Part model, mm, in its own coordinate system. Face numbers are marked on the shaded views. A direction names the side the tool comes from. Round coordinates to 2 decimals unless told otherwise and drop trailing zeros. Write each loop counter-clockwise with the first axis right and the second up, starting at its lowest first coordinate (ties: lowest second). Pieces come first, ordered by that corner, then holes. Notation, with made-up numbers: (40.5, -7.5) -> (77.5, -7.5) arc R22 cw to (77.5, 7.5) -> close; hole circle Ø5 at (69, -29). An arc over 180 degrees is marked (long way). Return JSON: item names as keys, results as strings. Group by question number.
(1) Drop flat-ended pins along their axis: pin 1 Ø2 at (x, z) = (7.5, -2) entering from -Y; pin 2 Ø8 at (x, y) = (6, 38.5) entering from -Z. Give the stop position or say it passes through.
(2) Tool access for the marked faces 1 and 2: list every direction of +Z, -Z, +X, -X, +Y, -Y with a clear straight run to the whole face (end or side of a thin tool).
(3) Saw through at B-B (x = 0). List the corners of the cut face in (y, z), plus the area to 3 significant figures.
(4) Mould opens along Y. For the marked faces 3, 4 and 5 say: +Y half, -Y half, draft (parallel to the pull), parting line (faces both ways), or undercut.
(5) Saw through at A-A (x = 7.5). State how many separate pieces and enclosed holes the cut face has, plus the area to 3 significant figures.
(6) Drill centre lines: L1, parallel to Y at x = 3, z = -3.25; L2, parallel to X at y = 5.5, z = -2; L3, parallel to Z at x = -7.5, y = 85.45. Where is each one in solid material? Low to high. Write a range as from..to.
(7) Saw through at D-D (y = 21). List the corners of the cut face in (x, z), plus the area to 3 significant figures.
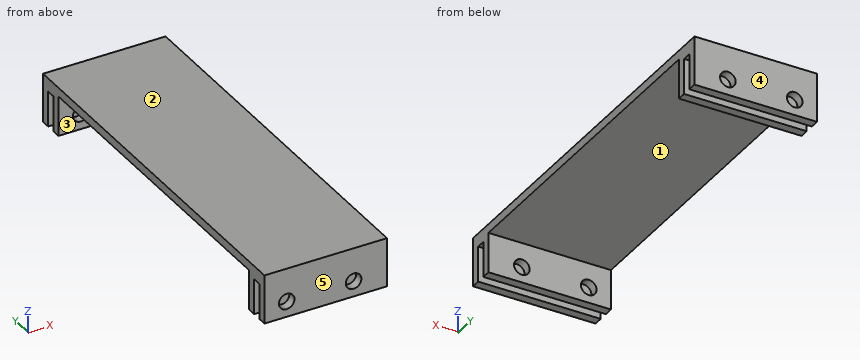
from build123d import *

# Parameters (mm, degrees)
SKETCH_1_W          = 30
SKETCH_1_H          = 11
EXTRUDE_1_DEPTH     = 6
SKETCH_2_W          = 16
SKETCH_2_H          = 2
CUT_EXTRUDE_1_DEPTH = 144
EXTRUDE_2_DEPTH     = 74
SKETCH_4_R          = 1.75
CUT_EXTRUDE_2_DEPTH = 144
SKETCH_5_W          = 11
SKETCH_5_H          = 80
CUT_EXTRUDE_3_DEPTH = 2.5
SKETCH_7_W          = 4
SKETCH_7_H          = 9
CUT_EXTRUDE_4_DEPTH = 74


with BuildPart() as part:
    # 草图1 → 凸台-拉伸1 (new body)
    with BuildSketch(Plane(origin=(0, 0, 0), x_dir=(1, 0, 0), z_dir=(0, 1, 0))):
        Rectangle(SKETCH_1_W, SKETCH_1_H)
    extrude_1 = extrude(amount=EXTRUDE_1_DEPTH)

    # 草图2 → 切除-拉伸1 (cut)
    with BuildSketch(Plane.ZY.offset(15)):
        with Locations((-5.5, 3)):
            Rectangle(SKETCH_2_W, SKETCH_2_H)
    cut_extrude_1 = extrude(amount=-CUT_EXTRUDE_1_DEPTH, mode=Mode.SUBTRACT)

    # 草图3 → 凸台-拉伸2 (add)
    with BuildSketch(Plane(origin=(0, 6, 0), x_dir=(1, 0, 0), z_dir=(0, 1, 0))):
        Polygon((2, 5.5), (-2, 5.5), (-2, -3.5), (-15, -3.5), (-15, -5.5), (15, -5.5), (15, -3.5), (2, -3.5), align=None)
    extrude(amount=EXTRUDE_2_DEPTH)

    # 草图4 → 切除-拉伸2 (cut)
    with BuildSketch(Plane(origin=(0, 6, 0), x_dir=(1, 0, 0), z_dir=(0, 1, 0))):
        with Locations(Location((-7.5, 2, 0), (0, 0, 270))):
            Circle(SKETCH_4_R)
        with Locations(Location((7.5, 2, 0), (0, 0, 270))):
            Circle(SKETCH_4_R)
    cut_extrude_2 = extrude(amount=-CUT_EXTRUDE_2_DEPTH, mode=Mode.SUBTRACT)

    # 草图5 → 切除-拉伸3 (cut)
    with BuildSketch(Plane.ZY.offset(15)):
        with Locations((0, 40)):
            Rectangle(SKETCH_5_W, SKETCH_5_H)
    cut_extrude_3 = extrude(amount=-CUT_EXTRUDE_3_DEPTH, mode=Mode.SUBTRACT)

    # 草图7 → 切除-拉伸4 (cut)
    with BuildSketch(Plane(origin=(0, 80, 0), x_dir=(1, 0, 0), z_dir=(0, 1, 0))):
        with Locations((0, 1)):
            Rectangle(SKETCH_7_W, SKETCH_7_H)
    extrude(amount=-CUT_EXTRUDE_4_DEPTH, mode=Mode.SUBTRACT)

    # 镜向1: 凸台-拉伸1, 切除-拉伸1, 切除-拉伸2, 切除-拉伸3 across plane
    add(extrude_1.mirror(Plane.ZX.offset(43)))
    add(cut_extrude_1.mirror(Plane.ZX.offset(43)), mode=Mode.SUBTRACT)
    add(cut_extrude_2.mirror(Plane.ZX.offset(43)), mode=Mode.SUBTRACT)
    add(cut_extrude_3.mirror(Plane.ZX.offset(43)), mode=Mode.SUBTRACT)


solid = part.part
Computed values:
{
 "1": {"pin 1": "through", "pin 2": "z = 3.5"},
 "2": {"face 1": "-Z, +X, -X", "face 2": "+Z, +X, -X, +Y, -Y"},
 "3": {"outline": "(0, -5.5) -> (2, -5.5) -> (2, 2.5) -> (4, 2.5) -> (4, -5.5) -> (6, -5.5) -> (6, 3.5) -> (80, 3.5) -> (80, -5.5) -> (82, -5.5) -> (82, 2.5) -> (84, 2.5) -> (84, -5.5) -> (86, -5.5) -> (86, 5.5) -> (0, 5.5) -> close", "area": "248 mm2"},
 "4": {"face 3": "undercut", "face 4": "+Y half", "face 5": "-Y half"},
 "5": {"separate pieces": "5", "enclosed holes": "0", "area": "220 mm2"},
 "6": {"L1": "0..2, 4..6, 80..82, 84..86", "L2": "-12.5..-9.25, -5.75..5.75, 9.25..15", "L3": "-5.5..-3.75, -0.25..5.5"},
 "7": {"outline": "(-12.5, 3.5) -> (15, 3.5) -> (15, 5.5) -> (-12.5, 5.5) -> close", "area": "55.0 mm2"}
}
